The drawing under review shows one solid part. Ordinate dimensions are in mm from its lowest x, y, z. Round coordinates to 2 decimals unless told otherwise and drop trailing zeros. Loops run counter-clockwise (first coordinate to the right, second up) from the corner with the lowest first, then second, coordinate; pieces in that order, holes last. Notation, with made-up numbers: M -40,86 L -10,86 A20 ccw -10,93 Z; hole C 8.5,68.5 d8. An arc over 180 degrees is marked long. Use a Markdown table: item, result.
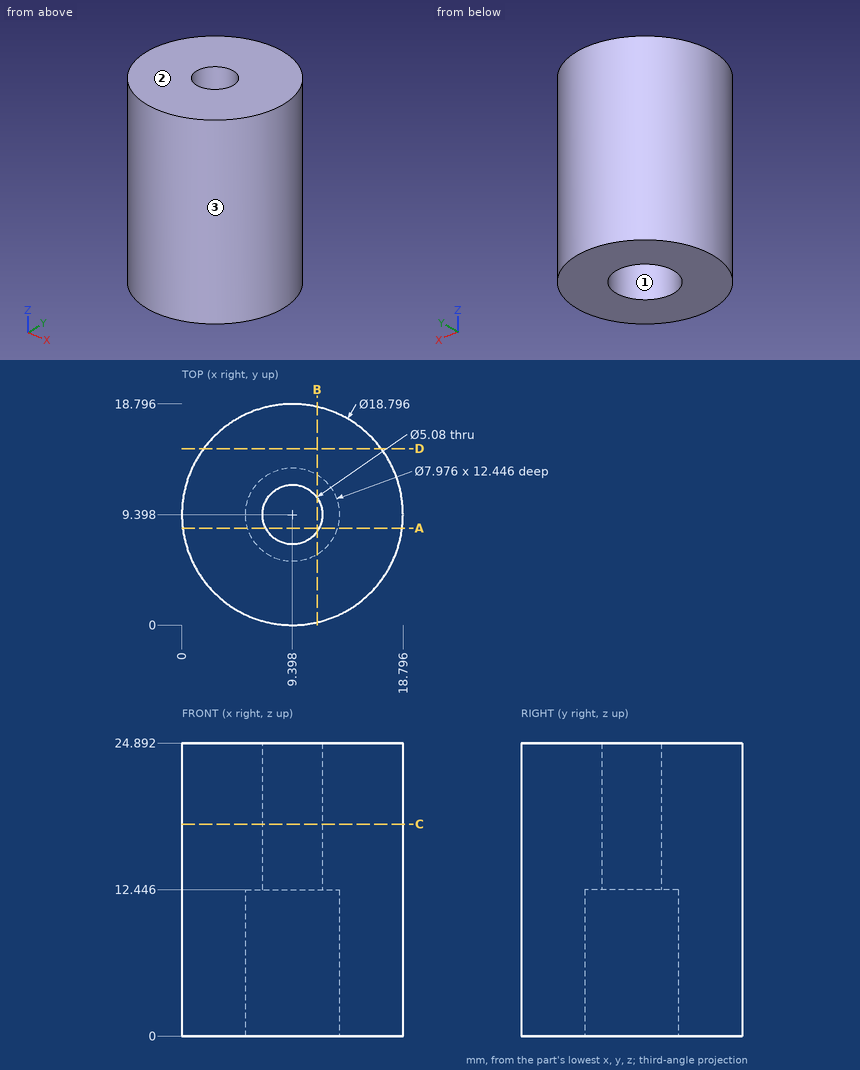
1. The part is to be moulded in two halves that separate along Y. For the marked faces 1, 2 and 3, say which applies: pulls with the +Y half, pulls with the -Y half, needs draft (parallel to the pull), parting line crosses it, or undercut.
Check values:
| item | result |
|---|---|
| face 1 | undercut |
| face 2 | needs draft |
| face 3 | parting line crosses it |
2. Wall thickness on line 1 along X through (y, z) = (9.75, 14.5); line 2 along Y through (x, z) = (5.75, 2.75) (1 decimal); line 3 along Z through (x, y) = (11.5, 11): over which ranges is each line inside the solid? List them lowest first. Write a range as from..to.
Check values:
| item | result |
|---|---|
| line 1 | x = 0.01..6.88, 11.91..18.79 |
| line 2 | y = 0.7..7.8, 11..18.1 |
| line 3 | z = 12.45..24.89 |
3. Take a section at B-B on x = 11.5. Give the boundary of the cut face in (y, z), and give its area (3 significant figures).
Check values:
| item | result |
|---|---|
| outline | M 0.24,0 L 6.01,0 L 6.01,12.45 L 7.97,12.45 L 7.97,24.89 L 0.24,24.89 Z; M 10.82,12.45 L 12.79,12.45 L 12.79,0 L 18.56,0 L 18.56,24.89 L 10.82,24.89 Z |
| area | 336 mm² |
4. Take a section at A-A on y = 8.25. Give the boundary of the cut face in (x, z) (1 decimal).
Check values:
| item | result |
|---|---|
| outline | M 0.1,0 L 5.6,0 L 5.6,12.4 L 7.1,12.4 L 7.1,24.9 L 0.1,24.9 Z; M 11.7,12.4 L 13.2,12.4 L 13.2,0 L 18.7,0 L 18.7,24.9 L 11.7,24.9 Z |
5. Take a section at D-D on y = 15. Give the boundary of the cut face in (x, z).
Check values:
| item | result |
|---|---|
| outline | M 1.85,0 L 16.94,0 L 16.94,24.89 L 1.85,24.89 Z |
6. Take a section at C-C on z = 18. Give the boundary of the cut face in (x, y), and give its area (3 significant figures).
Check values:
| item | result |
|---|---|
| outline | C 9.4,9.4 d18.8; hole C 9.4,9.4 d5.08 |
| area | 257 mm² |
7. Insertion check: pin 1 (4 mm diameter, centred on y = 7.5, z = 10, fed in from -X); pin 2 (4 mm diameter, centred on x = 9, y = 11, fed in from -Z); pin 3 (6 mm diameter, centred on x = 3.5, z = 13, fed in from -Y); pin 4 (2 mm diameter, centred on x = 7.5, z = 10.5, fed in from -Y). Each pin has a flat end and moves straight along its axis. Give the tip position at first contact, or say it passes through.
Check values:
| item | result |
|---|---|
| pin 1 | stops at x = 0 |
| pin 2 | stops at z = 12.45 |
| pin 3 | stops at y = 0.46 |
| pin 4 | stops at y = 0.04 |
